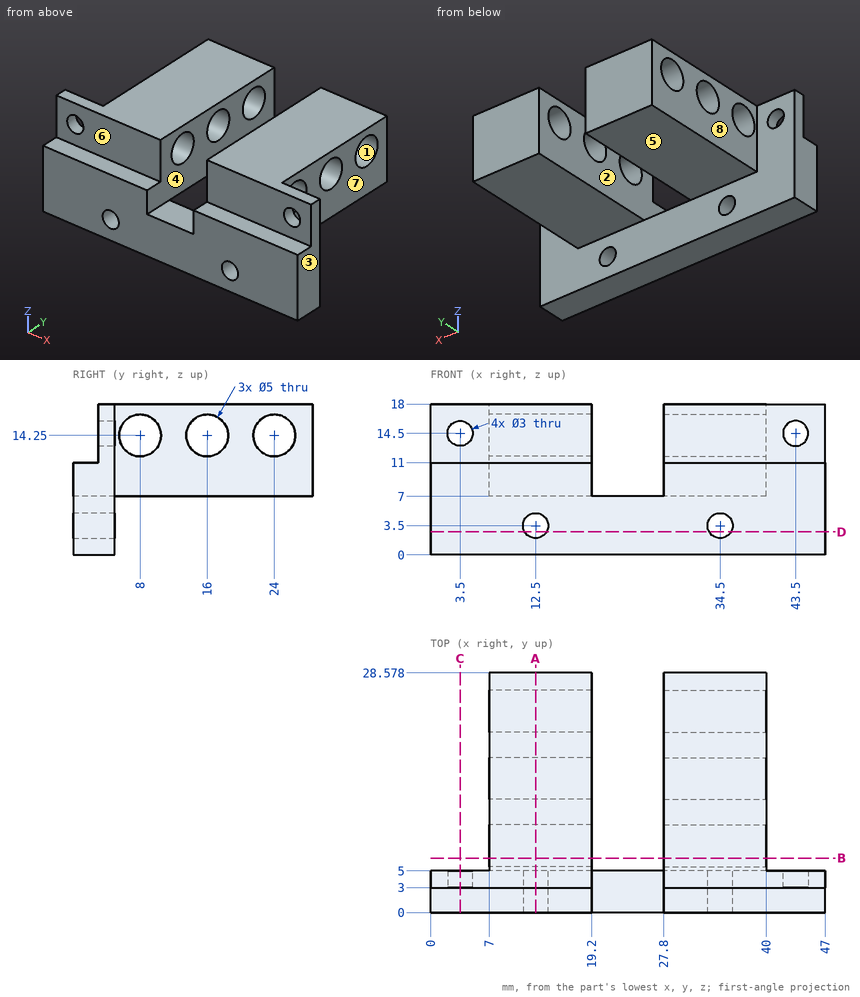
Source: three-view drawing plus pictorial views. Frame: mm from the lowest corner of the part. A direction names the side the tool comes from. Round coordinates to 2 decimals unless told otherwise and drop trailing zeros. Write each loop counter-clockwise with the first axis right and the second up, starting at its lowest first coordinate (ties: lowest second). Pieces come first, ordered by that corner, then holes. Notation, with made-up numbers: (-11.75, 66.5) -> (-4.75, 66.5) arc R27 cw to (-4.75, 98.5) -> close; hole circle Ø10 at (51.25, 89). An arc over 180 degrees is marked (long way). Return JSON: item names as keys, results as strings.
Q1. First-contact query: pin 1 Ø4 at (y, z) = (8, 14.25) entering from -X; pin 2 Ø3.5 at (x, z) = (3.5, 14.5) entering from -Y; pin 3 Ø10 at (x, y) = (11.5, 20.5) entering from -Z; pin 4 Ø9 at (y, z) = (13.5, 14.5) entering from -X. Flat tips, straight axial feed; report the tip coordinate or a pass-through.
From the geometry:
{"pin 1": "through", "pin 2": "y = 3", "pin 3": "z = 7", "pin 4": "x = 7"}
Q2. Set-up query: the marked faces 4, 5, 6, 7 and 8. Return all of +Z, -Z, +X, -X, +Y, -Y with unobstructed straight access to the full face (end or side cutting, diameter ignored); none if empty.
From the geometry:
{"face 4": "+Z, +Y, -Y", "face 5": "-Z, +X, -X, +Y", "face 6": "+Z, +X, -X, -Y", "face 7": "+Z, -Z, +X, +Y", "face 8": "+Z, -Z, -X, +Y"}
Q3. Section A-A on x = 12.5. Return the cut outline in (y, z).
From the geometry:
{"outline": "(0, 0) -> (5, 0) -> (5, 2) -> (0, 2) -> close; (0, 5) -> (5, 5) -> (5, 7) -> (28.58, 7) -> (28.58, 18) -> (3, 18) -> (3, 11) -> (0, 11) -> close; hole circle Ø5 at (8, 14.25); hole circle Ø5 at (16, 14.25); hole circle Ø5 at (24, 14.25)"}
Q4. Mould query, pull axis X, two halves, no side actions, for the marked faces 1, 2 and 3. Classes: +X half, -X half, draft (parallel to the pull), parting line (faces both ways), or undercut.
From the geometry:
{"face 1": "draft", "face 2": "undercut", "face 3": "+X half"}
Q5. Ray query, line 1 (Y direction, x = 12.25, z = 14.25); line 2 (Z direction, x = 43.5, y = 3.8); line 3 (X direction, y = 2.75, z = 10.75). Return the intervals inside material, ascending.
From the geometry:
{"line 1": "3 to 5.5, 10.5 to 13.5, 18.5 to 21.5, 26.5 to 28.58", "line 2": "0 to 13, 16 to 18", "line 3": "0 to 19.2, 27.8 to 47"}
Q6. Section B-B on y = 6.5. Return the cut outline in (x, z).
From the geometry:
{"outline": "(7, 7) -> (19.2, 7) -> (19.2, 12.25) -> (7, 12.25) -> close; (7, 16.25) -> (19.2, 16.25) -> (19.2, 18) -> (7, 18) -> close; (27.8, 7) -> (40, 7) -> (40, 12.25) -> (27.8, 12.25) -> close; (27.8, 16.25) -> (40, 16.25) -> (40, 18) -> (27.8, 18) -> close"}
Q7. Section C-C on x = 3.5. Return the cut outline in (y, z).
From the geometry:
{"outline": "(0, 0) -> (5, 0) -> (5, 13) -> (3, 13) -> (3, 11) -> (0, 11) -> close; (3, 16) -> (5, 16) -> (5, 18) -> (3, 18) -> close"}
Q8. Section D-D on z = 2.75. Return the cut outline in (x, y), and give its area (3 significant figures).
From the geometry:
{"outline": "(0, 0) -> (11.2, 0) -> (11.2, 5) -> (0, 5) -> close; (13.8, 0) -> (33.2, 0) -> (33.2, 5) -> (13.8, 5) -> close; (35.8, 0) -> (47, 0) -> (47, 5) -> (35.8, 5) -> close", "area": "209 mm2"}
